Input: part model. Units: mm. Frame: model coordinates. A direction names the side the tool comes from. Give positions to 0.01 mm unless a question says otherwise; leave off trailing zeros. Order: outer loops, then holes, each group sorted by start corner. A loop starts at its lowest first (then second) coordinate and runs counter-clockwise, first axis right, second up. Notation, with made-up numbers: (37.5, 85.5) - (79.5, 85.5) arc R20 cw to (79.5, 93.5) - close; hole circle Ø10 at (76, 31). An arc over 180 degrees is marked (long way). Answer in a Markdown table with one row per item. Add a question column.
from build123d import *

# Parameters (mm, degrees)
SKETCH1_W           = 304.8
SKETCH1_H           = 304.8
BOSS_EXTRUDE1_DEPTH = 2.54
SKETCH3_R           = 9.525
BOSS_EXTRUDE2_DEPTH = 12.7
SKETCH5_R           = 38.1
CUT_EXTRUDE2_DEPTH  = 255.31730181
SKETCH7_R           = 9.525
BOSS_EXTRUDE4_DEPTH = 53.0225
FILLET1_R           = 2.54
BOSS_EXTRUDE5_START = 31.75
SKETCH9_R           = 43.18
SKETCH9_R_2         = 38.1
BOSS_EXTRUDE5_DEPTH = 31.75


with BuildPart() as part:
    # Sketch1 → Boss-Extrude1 (new body)
    with BuildSketch(Plane(origin=(0, 0, 0), x_dir=(1, 0, 0), z_dir=(0, 1, 0))):
        with Locations((50.8, 0)):
            Rectangle(SKETCH1_W, SKETCH1_H)
    extrude(amount=BOSS_EXTRUDE1_DEPTH)

    # Sketch3 → Boss-Extrude2 (add)
    with BuildSketch(Plane(origin=(0, 2.54, 0), x_dir=(1, 0, 0), z_dir=(0, 1, 0))):
        with Locations(Location((57.15, 0, 0), (0, 0, 270))):
            Circle(SKETCH3_R)
    extrude(amount=BOSS_EXTRUDE2_DEPTH)

    # Sketch5 → Cut-Extrude2 (cut, through all)
    with BuildSketch(Plane(origin=(0, 2.54, 0), x_dir=(1, 0, 0), z_dir=(0, 1, 0))):
        with Locations(Location((-14.741985059, 0, 0), (0, 0, 270))):
            Circle(SKETCH5_R)
    extrude(amount=-CUT_EXTRUDE2_DEPTH, mode=Mode.SUBTRACT)

    # Sketch7 → Boss-Extrude4 (add)
    with BuildSketch(Plane(origin=(0, 2.54, 0), x_dir=(1, 0, 0), z_dir=(0, 1, 0))):
        with Locations(Location((-88.9, 76.2, 0), (0, 0, 90))):
            Circle(SKETCH7_R)
    boss_extrude4 = extrude(amount=BOSS_EXTRUDE4_DEPTH)

    # Mirror1: Boss-Extrude4 across plane
    add(boss_extrude4.mirror(Plane.XY))

    # Fillet1
    fillet1_edges = [part.edges().sort_by_distance(p)[0] for p in [
        (203.2, 1.27, 152.4),
    ]]
    fillet(fillet1_edges, radius=FILLET1_R)

    # Sketch9 → Boss-Extrude5 (add)
    with BuildSketch(Plane(origin=(0, 2.54, 0), x_dir=(1, 0, 0), z_dir=(0, 1, 0)).offset(BOSS_EXTRUDE5_START)):
        with Locations(Location((-14.741985059, 0, 0), (0, 0, 270))):
            Circle(SKETCH9_R)
        with Locations(Location((-14.741985059, 0, 0), (0, 0, 270))):
            Circle(SKETCH9_R_2, mode=Mode.SUBTRACT)
    extrude(amount=-BOSS_EXTRUDE5_DEPTH)


solid = part.part
Q1. Pull-direction query (X, two-part tool) for faces 4 (the cylindrical face through (-37.93, 17.39, -30.23)), 5 (the cylindrical face through (-80.45, 28.68, -80.6)), 6 (the cylindrical face through (47.85, 8.8, -2.06)), 7 (the flat face through (49, 0, -2)); classes: +X half, -X half, draft (parallel to the pull), parting line (faces both ways), or undercut.
Q2. Section D-D, the plane y = 42. Return loops of the section in (x, z) (3 decimals).
Q3. Line query: probe 1 along X at (y, z) = (14, 0) (3 decimals); probe 2 along X at (y, z) = (15.5, 0); probe 3 along X at (y, z) = (7, -3). Output: solid intervals per line, ascending.
Q4. Section C-C, the plane x = 57.15. Return loops of the section in (y, z) (3 decimals).
Q5. Contact query for flat-ended pins moving along their axis: P1, Ø5.5, axis at x = 60.5, z = 0, coming from the +Y side; P2, Ø3, axis at x = 135, z = 110, coming from the +Y side; P3, Ø4, axis at y = 15.5, z = 84.5, coming from the +X side. Output: stop coordinate, or through.
Q6. Section B-B, the plane x = -41.5. Return loops of the section in (y, z), then the cut area to 3 significant figures.
Q7. Section A-A, the plane z = 0. Return loops of the section in (x, y) (3 decimals).
Q8. Access query for faces 1 (the flat face through (57, 15.24, 0)), 2 (the cylindrical face through (-41.016, 18.637, -34.266)), 3 (the flat face through (-89, 55.562, -76)). Directions: +Z, -Z, +X, -X, +Y, -Y. A direction counts if a zero-diameter tool reaches every point of the face in a straight line with its end or side. Return the directions, or none.
Computed:
| question | item | result |
|---|---|---|
| 1 | face 4 | undercut |
| 1 | face 5 | parting line |
| 1 | face 6 | undercut |
| 1 | face 7 | draft |
| 2 | outline | circle Ø19.05 at (-88.9, -76.2); circle Ø19.05 at (-88.9, 76.2) |
| 3 | probe 1 | x = -57.922 to -52.842, 23.358 to 28.438, 47.625 to 66.675 |
| 3 | probe 2 | x = -57.92 to -52.84, 23.36 to 28.44 |
| 3 | probe 3 | x = -57.82 to -52.72, 23.24 to 28.33, 48.11 to 66.19 |
| 4 | outline | (0, -152.4) - (2.54, -152.4) - (2.54, -9.525) - (15.24, -9.525) - (15.24, 9.525) - (2.54, 9.525) - (2.54, 152.4) - (0, 152.4) - close |
| 5 | P1 | stops at y = 15.24 |
| 5 | P2 | stops at y = 2.54 |
| 5 | P3 | stops at x = -81.76 |
| 6 | outline | (0, -152.4) - (2.54, -152.4) - (2.54, -33.89) - (34.29, -33.89) - (34.29, -27.12) - (0, -27.12) - close; (0, 27.12) - (34.29, 27.12) - (34.29, 33.89) - (2.54, 33.89) - (2.54, 152.4) - (0, 152.4) - close |
| 6 | area | 1,070 mm^2 |
| 7 | outline | (-101.6, 0) - (-52.842, 0) - (-52.842, 34.29) - (-57.922, 34.29) - (-57.922, 2.54) - (-101.6, 2.54) - close; (23.358, 0) - (203.2, 0) - (203.2, 2.54) - (66.675, 2.54) - (66.675, 15.24) - (47.625, 15.24) - (47.625, 2.54) - (28.438, 2.54) - (28.438, 34.29) - (23.358, 34.29) - close |
| 8 | face 1 | +Z, -Z, +X, +Y |
| 8 | face 2 | +Y |
| 8 | face 3 | +Z, -Z, +X, -X, +Y |
